Check sheet for the modelled part. Datum: model origin and axes. Units: mm. A direction names the side the tool comes from. Round coordinates to 2 decimals unless told otherwise and drop trailing zeros. Order: outer loops, then holes, each group sorted by start corner. A loop starts at its lowest first (then second) coordinate and runs counter-clockwise, first axis right, second up.
Q1. Mould release check, pull along X, two halves, no side actions. Record for faces 1 (the cylindrical face through (0.783, 13.688, 162.717)), 2 (the flat face through (0, 20, 88)), 3 (the flat face through (1.588, 20, 88)), 4 (the flat face through (13, 49.212, 88)): +X half, -X half, draft (parallel to the pull), parting line (faces both ways), or undercut.
Q2. Cross-section at A-A on z = 139.7. Record the cut outline in (x, y).
Q3. Cross-section at B-B on x = 12.25. Record the cut outline in (y, z).
Q4. Set-up check for faces 5 (the flat face through (23.812, 30, 88)), 6 (the cylindrical face through (24.595, 37.987, 40.677)): record each of +Z, -Z, +X, -X, +Y, -Y from which the full face is reachable in a straight line by a thin tool's end or side.
Q5. Scan lines: probe 1 along Y at (x, z) = (1, 12.7); probe 2 along Y at (x, z) = (10.5, 115.5); probe 3 along X at (y, z) = (30.5, 71). Record each from-to range of solid material in increasing order.
Q6. Cross-section at C-C on z = 38.1. Record the cut outline in (x, y), then the cut area to 3 significant figures.
Q7. Cross-section at D-D on y = 43. Record the cut outline in (x, z).
Autodesk Inventor part; units mm, degrees
ref_plane "YZ Plane" through (0, 0, 0) normal (1, 0, 0) x (0, 1, 0)
ref_plane "XZ Plane" through (0, 0, 0) normal (0, 1, 0) x (-1, 0, 0)
ref_plane "XY Plane" through (0, 0, 0) normal (0, 0, 1) x (1, 0, 0)
sketch "Sketch1" plane through (0, 0, 0) normal (0, 0, 1) x (1, 0, 0)
  line L0 (0, 0) -> (25.4, 0)
  line L1 (25.4, 0) -> (25.4, 50.8)
  line L2 (25.4, 50.8) -> (0, 50.8)
  line L3 (0, 50.8) -> (0, 0)
  dimension "d0" = 25.4
  dimension "d1" = 50.8
extrude "Extrusion1" add sketch "Sketch1" along normal blind 177.8
shell "Shell1" thickness 1.5875 removed faces 2 at (8.4667, 16.9333, 0) at (8.4667, 16.9333, 177.8)
hole "Hole1" at (25.4, 25.4, 114.3) direction (-1, 0, 0) diameter 28.575 end through all
sketch "Sketch2" plane through (25.4, 0, 0) normal (1, 0, 0) x (0, 0, -1)
  line L0 (-177.8, 1.5875) -> (-177.8, 49.2125)
  line L1 (-177.8, 25.4) -> (-114.3, 25.4)
  line L2 (-177.8, 25.4) -> (-114.3, 25.4) construction
  line L3 (-114.3, 25.4) -> (-88.9, 25.4)
  line L4 (-114.3, 25.4) -> (-139.7, 25.4)
  circle A0 centre (-139.7, 25.4) radius 2.5797
  circle A1 centre (-88.9, 25.4) radius 2.5797
  point P0 (0, 0)
  dimension "d14" = 63.5
  dimension "d16" = 25.4
  dimension "d17" = 25.4
  dimension "d18" = 5.1594
  dimension "d19" = 5.1594
extrude "Extrusion2" cut sketch "Sketch2" against normal blind 177.8
hole "Hole2" at (25.4, 38.1, 165.1) direction (-1, 0, 0) diameter 5.1594 end through all
hole "Hole3" at (25.4, 12.7, 165.1) direction (-1, 0, 0) diameter 5.1594 end through all
hole "Hole4" at (25.4, 38.1, 12.7) direction (-1, 0, 0) diameter 5.1594 end through all
hole "Hole5" at (25.4, 38.1, 38.1) direction (-1, 0, 0) diameter 5.1594 end through all
hole "Hole6" at (25.4, 12.7, 38.1) direction (-1, 0, 0) diameter 5.1594 end through all
hole "Hole7" at (25.4, 12.7, 12.7) direction (-1, 0, 0) diameter 5.1594 end through all
properties part number "1x2 7 in Beam Motor Mount"
Results found:
1. face 1: draft
1. face 2: -X half
1. face 3: undercut
1. face 4: undercut
2. outline: (0, 0) - (25.4, 0) - (25.4, 22.82) - (23.81, 22.82) - (23.81, 1.59) - (1.59, 1.59) - (1.59, 22.82) - (0, 22.82) - close; (0, 27.98) - (1.59, 27.98) - (1.59, 49.21) - (23.81, 49.21) - (23.81, 27.98) - (25.4, 27.98) - (25.4, 50.8) - (0, 50.8) - close
3. outline: (0, 0) - (1.59, 0) - (1.59, 177.8) - (0, 177.8) - close; (49.21, 0) - (50.8, 0) - (50.8, 177.8) - (49.21, 177.8) - close
4. face 5: +Z, -Z
4. face 6: +X, -X
5. probe 1: y = 0 to 10.12, 15.28 to 35.52, 40.68 to 50.8
5. probe 2: y = 0 to 1.59, 49.21 to 50.8
5. probe 3: x = 0 to 1.59, 23.81 to 25.4
6. outline: (0, 0) - (25.4, 0) - (25.4, 10.12) - (23.81, 10.12) - (23.81, 1.59) - (1.59, 1.59) - (1.59, 10.12) - (0, 10.12) - close; (0, 15.28) - (1.59, 15.28) - (1.59, 35.52) - (0, 35.52) - close; (0, 40.68) - (1.59, 40.68) - (1.59, 49.21) - (23.81, 49.21) - (23.81, 40.68) - (25.4, 40.68) - (25.4, 50.8) - (0, 50.8) - close; (23.81, 15.28) - (25.4, 15.28) - (25.4, 35.52) - (23.81, 35.52) - close
6. area: 199 mm2
7. outline: (0, 0) - (1.59, 0) - (1.59, 177.8) - (0, 177.8) - close; (23.81, 0) - (25.4, 0) - (25.4, 177.8) - (23.81, 177.8) - close
